The model under review builds one solid part; all positions refer to its coordinate system, in mm. Coordinates: 2 decimals unless noted, no trailing zeros. Loops run counter-clockwise (first coordinate to the right, second up) from the corner with the lowest first, then second, coordinate; pieces in that order, holes last. Notation, with made-up numbers: M -12,62 L -7,62 A20 ccw -7,94 Z; hole C -23,-28 d9. An arc over 180 degrees is marked long. Return JSON: item names as keys, results as strings.
```python
from build123d import *

# Parameters (mm, degrees)
SKETCH1_W           = 203.2
SKETCH1_H           = 76.2
BOSS_EXTRUDE1_DEPTH = 133.35
SHELL1_T            = -6.35
SKETCH2_W           = 1.5875
SKETCH2_H           = 72.39
CUT_EXTRUDE1_DEPTH  = 127
LPATTERN1_COUNT     = 13
LPATTERN1_PITCH     = 12.7
CUT_EXTRUDE2_START  = -127
SKETCH3_W           = 1.5875
SKETCH3_H           = 72.39
CUT_EXTRUDE2_DEPTH  = 127


with BuildPart() as part:
    # Sketch1 → Boss-Extrude1 (new body)
    with BuildSketch(Plane.XY):
        Rectangle(SKETCH1_W, SKETCH1_H)
    extrude(amount=BOSS_EXTRUDE1_DEPTH)

    # Shell1
    shell1_openings = [part.faces().sort_by_distance(p)[0] for p in [
        (0, 0, 133.35),
    ]]
    offset(amount=SHELL1_T, openings=shell1_openings, kind=Kind.INTERSECTION)

    # Sketch2 → Cut-Extrude1 (cut)
    with BuildSketch(Plane.XY.offset(133.35)):
        with Locations((-91.28125, 0)):
            Rectangle(SKETCH2_W, SKETCH2_H)
    cut_extrude1 = extrude(amount=-CUT_EXTRUDE1_DEPTH, mode=Mode.SUBTRACT)

    # LPattern1: Cut-Extrude1 ×13
    with Locations(*[(i * LPATTERN1_PITCH, 0, 0) for i in range(1, LPATTERN1_COUNT)]):
        add(cut_extrude1, mode=Mode.SUBTRACT)

    # Sketch3 → Cut-Extrude2 (cut)
    with BuildSketch(Plane.XY.offset(133.35).offset(CUT_EXTRUDE2_START)):
        with Locations((88.33739, 0)):
            Rectangle(SKETCH3_W, SKETCH3_H)
    extrude(amount=CUT_EXTRUDE2_DEPTH, mode=Mode.SUBTRACT)


solid = part.part
```
1. To check wall thickness, follow line 1 (Y direction, x = -60, z = 116); line 2 (Y direction, x = 11, z = 64.5) (3 decimals); line 3 (X direction, y = 24.5, z = 70). State the ranges of each line that lie inside material, in increasing order.
Check values:
{"line 1": "-38.1 to -31.75, 31.75 to 38.1", "line 2": "-38.1 to -36.195, 36.195 to 38.1", "line 3": "-101.6 to -95.25, 95.25 to 101.6"}
2. Add section B-B on y = 18. Give the boundary of the cut face in (x, z).
Check values:
{"outline": "M -101.6,0 L 101.6,0 L 101.6,133.35 L 95.25,133.35 L 95.25,6.35 L -95.25,6.35 L -95.25,133.35 L -101.6,133.35 Z"}
3. Add section A-A on x = -24. Give the boundary of the cut face in (y, z), plus the area to 3 significant figures.
Check values:
{"outline": "M -38.1,0 L 38.1,0 L 38.1,133.35 L 31.75,133.35 L 31.75,6.35 L -31.75,6.35 L -31.75,133.35 L -38.1,133.35 Z", "area": "2,100 mm²"}
4. Insertion check: pin 1 Ø1.5 at (x, y) = (-65, -20.5) entering from +Z. The pin has a flat end and moves straight along its axis. Give the tip position at first contact, or say it passes through.
Check values:
{"pin 1": "z = 6.35"}
5. The part is to be moulded in two halves that separate along X. For faces 1 (the face through (101.6, -1, 66)), 2 (the face through (0, 34, 133.35)), 3 (the face through (9.525, -34, 71)), say which applies: released by +X, released by -X, zero draft, split by the parting line, or undercut.
Check values:
{"face 1": "released by +X", "face 2": "zero draft", "face 3": "undercut"}
